from build123d import *

# Parameters (mm, degrees)
F0_R     = 7
F1_DEPTH = 4.4
F3_DEPTH = 2.6
F6_R     = 4
F7_DEPTH = 12


with BuildPart() as f1:
    # F0 (on Top) → F1 (new body)
    with BuildSketch(Plane.XY):
        Circle(F0_R)
    extrude(amount=F1_DEPTH)

    # F2 (on face) → F3 (cut)
    with BuildSketch(Plane.XY.offset(4.4)):
        Polygon((2.5, -1.443376), (2.5, 1.443376), (0, 2.886751), (-2.5, 1.443376), (-2.5, -1.443376), (0, -2.886751), align=None)
    extrude(amount=-F3_DEPTH, mode=Mode.SUBTRACT)

    # F4 (on Right) → F5 (revolve, cut)
    with BuildSketch(Plane.YZ):
        with BuildLine():
            Line((-7, 4.4), (-7, 0))
            ThreePointArc((-7, 0), (-6.319513, 2.483371), (-4.6, 4.4))
            Line((-4.6, 4.4), (-7, 4.4))
        make_face()
    revolve(axis=Axis((0, 0, 2.2), (0, 0, 1)), mode=Mode.SUBTRACT)

    # F6 (on Top) → F7 (join)
    with BuildSketch(Plane.XY):
        Circle(F6_R)
    extrude(amount=-F7_DEPTH)


solid = f1.part
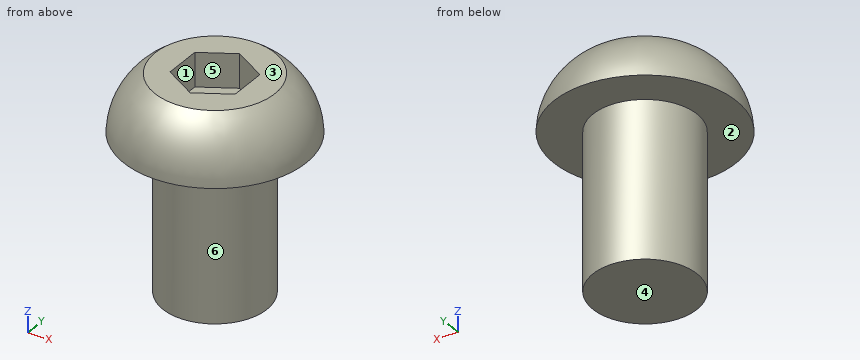
Geometry: final body of the model. Coordinates: model frame, mm. Face numbers are marked on the shaded views. A direction names the side the tool comes from. Give positions to 0.01 mm unless a question says otherwise; leave off trailing zeros. Write each loop counter-clockwise with the first axis right and the second up, starting at its lowest first coordinate (ties: lowest second). Pieces come first, ordered by that corner, then holes.
(1) Cut plane A-A, the plane z = -5.5. Return loops of the section in (x, y), then the cut area to 3 significant figures.
(2) Ray query, line 1 (X direction, y = -1.25, z = 2.5); line 2 (X direction, y = 0, z = 3.25); line 3 (Z direction, x = -2, y = -3.5). Return the intervals inside material, ascending.
(3) Access query for the marked faces 1, 2 and 3. Directions: +Z, -Z, +X, -X, +Y, -Y. A direction counts if a zero-diameter tool reaches every point of the face in a straight line with its end or side. Return the directions, or none.
(4) First-contact query: P1, Ø8, axis at y = 5, z = -4.5, coming from the -X side; P2, Ø1.5, axis at y = 0, z = -6.5, coming from the -X side; P3, Ø3, axis at y = 0.5, z = 3, coming from the +X side. Flat tips, straight axial feed; report the tip coordinate or a pass-through.
(5) Mould query, pull axis Y, two halves, no side actions, for the marked faces 4, 5 and 6. Classes: released by +Y, released by -Y, zero draft, split by the parting line, or undercut.
Values follow:
1. outline: circle Ø8 at (0, 0)
1. area: 50.3 mm2
2. line 1: x = -6.19 to -2.5, 2.5 to 6.19
2. line 2: x = -5.82 to -2.5, 2.5 to 5.82
2. line 3: z = 0 to 4.4
3. face 1: +Z
3. face 2: -Z
3. face 3: +Z, +X, -X, +Y, -Y
4. P1: stops at x = -3.87
4. P2: stops at x = -4
4. P3: stops at x = 6.73
5. face 4: zero draft
5. face 5: undercut
5. face 6: split by the parting line
